Part model, mm, in its own coordinate system. Face numbers are marked on the shaded views. A direction names the side the tool comes from. Give positions to 0.01 mm unless a question says otherwise; leave off trailing zeros. Order: outer loops, then holes, each group sorted by start corner. A loop starts at its lowest first (then second) coordinate and runs counter-clockwise, first axis right, second up. Notation, with made-up numbers: (31, -22) - (67, -22) arc R26 ccw to (67, 17) - close; hole circle Ø6 at (79.5, -0.75). An arc over 180 degrees is marked (long way). Use a Markdown table: item, result. Add a question column.
from build123d import *

# Parameters (mm, degrees)
CROQUIS2_R              = 8
SALIENTE_EXTRUIR1_DEPTH = 2
CROQUIS3_R              = 7
CORTAR_EXTRUIR1_DEPTH   = 1
CROQUIS4_R              = 6
CROQUIS5_R              = 3.5
CROQUIS6_R              = 3.5
SALIENTE_EXTRUIR2_DEPTH = 4
CROQUIS9_R              = 3.5
CROQUIS10_R             = 5.916
CROQUIS11_R             = 6.5
SALIENTE_EXTRUIR3_DEPTH = 3.5
REDONDEO2_R             = 1
CROQUIS15_R             = 5.88
SALIENTE_EXTRUIR4_DEPTH = 0.001
C_PULA1_FACE_RADIUS     = 5.88
C_PULA1_HEIGHT          = 3
CROQUIS16_R             = 1.4
CORTAR_EXTRUIR2_DEPTH   = 6


with BuildPart() as part:
    # Croquis2 → Saliente-Extruir1 (new body)
    with BuildSketch(Plane.XY):
        Circle(CROQUIS2_R)
    extrude(amount=SALIENTE_EXTRUIR1_DEPTH)

    # Croquis3 → Cortar-Extruir1 (cut)
    with BuildSketch(Plane.XY.offset(2)):
        Circle(CROQUIS3_R)
    extrude(amount=-CORTAR_EXTRUIR1_DEPTH, mode=Mode.SUBTRACT)

    # Croquis4 → Recubrir1 section 0
    with BuildSketch(Plane.XY.offset(1)):
        Circle(CROQUIS4_R)
    # Croquis5 → Recubrir1 section 1
    with BuildSketch(Plane.XY.offset(2.5)):
        Circle(CROQUIS5_R)
    loft()

    # Croquis6 → Saliente-Extruir2 (add)
    with BuildSketch(Plane.XY.offset(2.5)):
        Circle(CROQUIS6_R)
    extrude(amount=SALIENTE_EXTRUIR2_DEPTH)

    # Croquis9 → Recubrir3 section 0
    with BuildSketch(Plane.XY.offset(6.5)):
        Circle(CROQUIS9_R)
    # Croquis10 → Recubrir3 section 1
    with BuildSketch(Plane.XY.offset(7.952)):
        Circle(CROQUIS10_R)
    loft()

    # Croquis11 → Saliente-Extruir3 (add)
    with BuildSketch(Plane.XY.offset(7.952)):
        Circle(CROQUIS11_R)
    extrude(amount=SALIENTE_EXTRUIR3_DEPTH)

    # Redondeo2
    # the kernel refuses this fillet: 1 mm, written as the material it takes off along each edge
    with BuildSketch(Plane(origin=(0, 0, 7.952), x_dir=(1, 0, 0), z_dir=(0, -1, 0))) as redondeo2_piece_1:
        with BuildLine():
            CenterArc((5.5, 0.909364613), REDONDEO2_R, 294.582307044, 65.417692956)
            Line((5.916, 0), (5.92432, -0.018187292))
            ThreePointArc((5.92432, -0.018187292), (6.208, -0.02), (6.5, -0.02))
            Line((6.5, -0.02), (6.52, 0))
            Line((6.52, 0), (6.52, 0.909364613))
            Line((6.52, 0.909364613), (6.5, 0.909364613))
        make_face()
    revolve(axis=Axis((0, 0, 7.952), (0, 0, 1)), mode=Mode.SUBTRACT)

    # Croquis15 → Saliente-Extruir4 (add)
    with BuildSketch(Plane.XY.offset(11.452)):
        Circle(CROQUIS15_R)
    extrude(amount=SALIENTE_EXTRUIR4_DEPTH)

    # Cúpula1: a dome of height H over a round flat face of radius A is a cap of a sphere of radius (A * A + H * H) / (2 * H)
    c_pula1_r = (C_PULA1_FACE_RADIUS * C_PULA1_FACE_RADIUS + C_PULA1_HEIGHT * C_PULA1_HEIGHT) / (2 * C_PULA1_HEIGHT)
    c_pula1_base = Plane((0, 0, 11.453), z_dir=(0, 0, 1))
    with Locations(c_pula1_base.offset(C_PULA1_HEIGHT - c_pula1_r)):
        c_pula1_ball = Sphere(c_pula1_r, mode=Mode.PRIVATE)
    add(split(c_pula1_ball, bisect_by=c_pula1_base, keep=Keep.TOP, mode=Mode.PRIVATE))

    # Croquis16 → Cortar-Extruir2 (cut)
    with BuildSketch(Plane(origin=(0, 0, 0), x_dir=(-1, 0, 0), z_dir=(0, 0, -1))):
        Circle(CROQUIS16_R)
    extrude(amount=-CORTAR_EXTRUIR2_DEPTH, mode=Mode.SUBTRACT)


solid = part.part
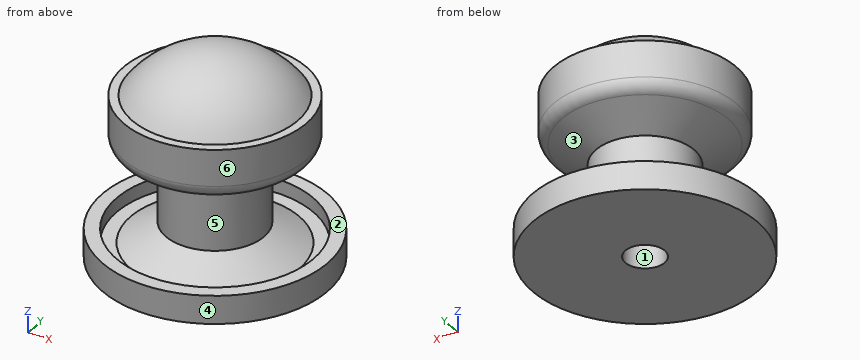
1. Tool access for the marked faces 4, 5 and 6: list every direction of +Z, -Z, +X, -X, +Y, -Y with a clear straight run to the whole face (end or side of a thin tool).
2. Cut at C-C (z = 1.5). Write the cut outline in (x, y).
3. Pin check, flat tips, straight feed: P1, Ø1, axis at x = 0.5, y = 0, coming from the +Z side; P2, Ø5, axis at x = 3.5, y = 3.5, coming from the +Z side; P3, Ø1.5, axis at x = -5.5, y = 5, coming from the +Z side; P4, Ø6, axis at x = 6, z = 7.5, coming from the -Y side. Stop position of each tip, or through.
4. Drill centre lines: probe 1 along Y at (x, z) = (0, 1.65); probe 2 along Y at (x, z) = (0, 4); probe 3 along Y at (x, z) = (0, 1.55). Where is each one in solid material? Low to high. Write a range as [from, to].
5. Cut at B-B (z = 3.5). Write the cut outline in (x, y).
6. Mould opens along Z. For the marked faces 1, 2 and 3 say: released by +Z, released by -Z, zero draft, split by the parting line, or undercut.
7. Cut at D-D (z = 12.5). Write the cut outline in (x, y).
Responses:
| question | item | result |
|---|---|---|
| 1 | face 4 | +Z, -Z |
| 1 | face 5 | none |
| 1 | face 6 | +Z |
| 2 | outline | circle Ø16 at (0, 0); circle Ø10.33 at (0, 0); hole circle Ø14 at (0, 0); hole circle Ø2.8 at (0, 0) |
| 3 | P1 | stops at z = 14.45 |
| 3 | P2 | stops at z = 14.03 |
| 3 | P3 | stops at z = 2 |
| 3 | P4 | stops at y = -5.62 |
| 4 | probe 1 | y = [-8, -7], [-4.92, -1.4], [1.4, 4.92], [7, 8] |
| 4 | probe 2 | y = [-3.5, -1.4], [1.4, 3.5] |
| 4 | probe 3 | y = [-8, -7], [-5.08, -1.4], [1.4, 5.08], [7, 8] |
| 5 | outline | circle Ø7 at (0, 0); hole circle Ø2.8 at (0, 0) |
| 6 | face 1 | zero draft |
| 6 | face 2 | released by +Z |
| 6 | face 3 | undercut |
| 7 | outline | circle Ø9.91 at (0, 0) |
